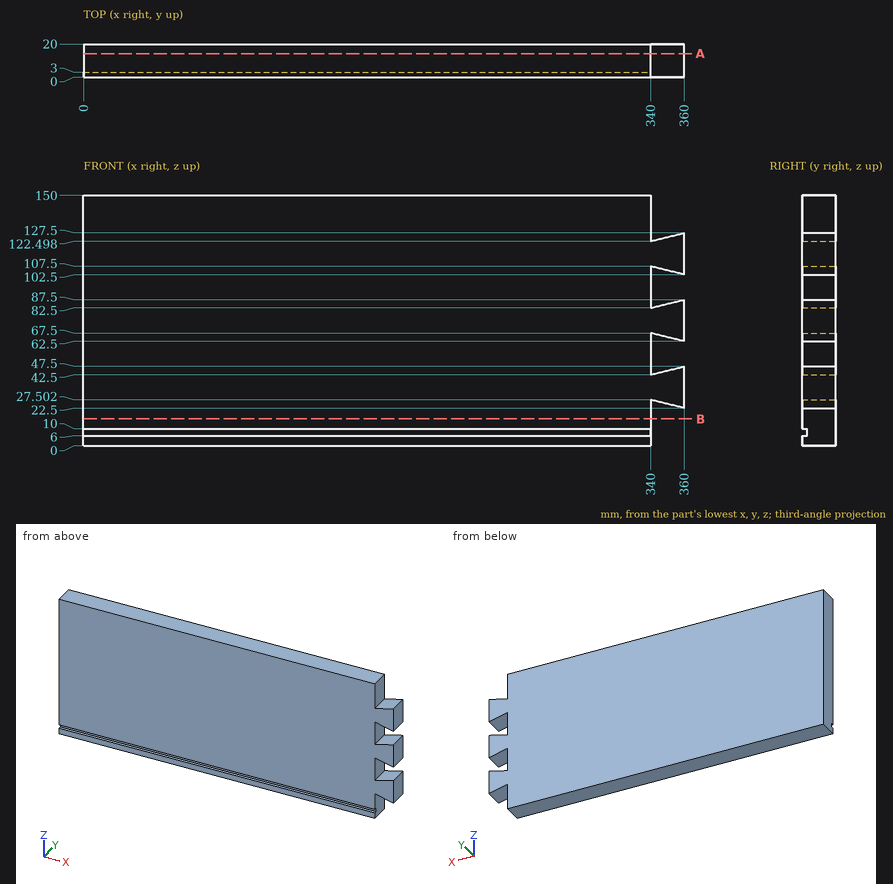
Drawing for the job (mm, zero at the part's lowest x, y, z). Give positions to 0.01 mm unless a question says otherwise; leave off trailing zeros. Order: outer loops, then holes, each group sorted by start corner. A loop starts at its lowest first (then second) coordinate and runs counter-clockwise, first axis right, second up. Notation, with made-up numbers: M -11,89 L -5,89 A17 cw -5,117 Z; hole C 73,6 d2. An arc over 180 degrees is marked long. Use a Markdown table: item, result. Add a question column.
(1) Saw through at B-B, the plane z = 16. Give the cut face in (x, y), and give its area (3 significant figures).
(2) Saw through at A-A, the plane y = 14.25. Give the cut face in (x, z), and give its area (3 significant figures).
(3) Probe line 1 along X through (y, z) = (12.5, 141.5). List the from-to ranges inside material, lowest first. Write a range as [from, to].
Answer key:
| question | item | result |
|---|---|---|
| 1 | outline | M 0,0 L 340,0 L 340,20 L 0,20 Z |
| 1 | area | 6,800 mm^2 |
| 2 | outline | M 0,0 L 340,0 L 340,27.5 L 360,22.5 L 360,47.5 L 340,42.5 L 340,67.5 L 360,62.5 L 360,87.5 L 340,82.5 L 340,107.5 L 360,102.5 L 360,127.5 L 340,122.5 L 340,150 L 0,150 Z |
| 2 | area | 52,200 mm^2 |
| 3 | line 1 | [0, 340] |
